from build123d import *

# Parameters (mm, degrees)
BASIC_SHAPE_DEPTH              = 4.9
SIDE_PROFILE1_DEPTH            = 4.55
SIDE_PROFILE1_DEPTH_BACK       = 4.55
SIDE_PROFILE2_DEPTH            = 4.55
SIDE_PROFILE2_DEPTH_BACK       = 4.55
LOCATION_MARK_DEPTH            = 0.8
SKETCH6_W                      = 0.25
SKETCH6_H                      = 1.39
PIN_RELIEF_DEPTH               = 1.25
REMAINING_PINS_COUNT           = 4
REMAINING_PINS_PITCH           = 2.54
REMAINING_PINS_COPY_1_SKETCH_W = 0.25
REMAINING_PINS_COPY_1_SKETCH_H = 1.39
REMAINING_PINS_COPY_2_SKETCH_W = 0.25
REMAINING_PINS_COPY_2_SKETCH_H = 1.39
REMAINING_PINS_COPY_3_SKETCH_W = 0.25
REMAINING_PINS_COPY_3_SKETCH_H = 1.39
REMAINING_PINS_COPY_4_DEPTH    = 1.25
REMAINING_PINS_COPY_5_DEPTH    = 1.25
REMAINING_PINS_COPY_6_DEPTH    = 1.25
PIN_SHAPE1_DEPTH               = 0.445
PIN_START                      = -0.445
PIN_SHAPE2_DEPTH               = 0.445


with BuildPart() as part:
    # Sketch1 → Basic Shape (new body, symmetric)
    with BuildSketch(Plane(origin=(0, 0, 0), x_dir=(1, 0, 0), z_dir=(0, 1, 0))):
        Polygon((-3.3, -0.7), (-3.55, -2.75), (-3.3, -4.8), (3.3, -4.8), (3.55, -2.75), (3.3, -0.7), align=None)
    extrude(amount=BASIC_SHAPE_DEPTH, both=True)

    # Sketch2 → Side Profile1 (cut, two sides)
    with BuildSketch(Plane(origin=(0, 0, 0), x_dir=(0, 0, -1), z_dir=(1, 0, 0))) as side_profile1_sk:
        Polygon((-4.8, 4.9), (-4.8, 4.65), (-2.75, 4.9), align=None)
        Polygon((-4.8, -4.9), (-2.75, -4.9), (-4.8, -4.65), align=None)
    extrude(amount=SIDE_PROFILE1_DEPTH, mode=Mode.SUBTRACT)
    extrude(side_profile1_sk.sketch, amount=-SIDE_PROFILE1_DEPTH_BACK, mode=Mode.SUBTRACT)

    # Sketch3 → Side Profile2 (cut, two sides)
    with BuildSketch(Plane(origin=(0, 0, 0), x_dir=(0, 0, -1), z_dir=(1, 0, 0))) as side_profile2_sk:
        Polygon((-2.75, 4.9), (-0.7, 4.9), (-0.7, 4.65), align=None)
        Polygon((-2.75, -4.9), (-0.7, -4.9), (-0.7, -4.65), align=None)
    extrude(amount=SIDE_PROFILE2_DEPTH, mode=Mode.SUBTRACT)
    extrude(side_profile2_sk.sketch, amount=-SIDE_PROFILE2_DEPTH_BACK, mode=Mode.SUBTRACT)

    # Sketch4 → Location Mark (cut)
    with BuildSketch(Plane(origin=(0, 0, 4.8), x_dir=(-1, 0, 0), z_dir=(0, 0, -1))):
        with BuildLine():
            Line((0.7, 4.65), (0.7, 3.45))
            ThreePointArc((0.7, 3.45), (0, 2.75), (-0.7, 3.45))
            Line((-0.7, 3.45), (-0.7, 4.65))
            Line((-0.7, 4.65), (0.7, 4.65))
        make_face()
    extrude(amount=LOCATION_MARK_DEPTH, mode=Mode.SUBTRACT)

    # First Pin: sweep along a path in Sketch5
    with BuildLine(Plane(origin=(0, -3.9, 0), x_dir=(1, 0, 0), z_dir=(0, 1, 0))) as first_pin_path:
        Line((0, -2.75), (3.31, -2.75))
        ThreePointArc((3.31, -2.75), (3.663553391, -2.603553391), (3.81, -2.25))
        Line((3.81, -2.25), (3.81, 3.3))
    # Sketch6 → First Pin (sweep)
    with BuildSketch(Plane(origin=(0, 0, 0), x_dir=(0, 0, -1), z_dir=(1, 0, 0))):
        with Locations((-2.75, -3.9)):
            Rectangle(SKETCH6_W, SKETCH6_H)
    first_pin = sweep(path=first_pin_path.line)

    # Sketch7 → Pin Relief (cut, through all)
    with BuildSketch(Plane.ZY.offset(-3.685)):
        Polygon((-3.3, -4.15), (0, -4.15), (0, -4.3725), (0.7, -4.595), (-3.3, -4.595), align=None)
        Polygon((-3.3, -3.65), (0, -3.65), (0, -3.4275), (0.7, -3.205), (-3.3, -3.205), align=None)
    pin_relief = extrude(amount=-PIN_RELIEF_DEPTH, mode=Mode.SUBTRACT)

    # Opp Pin: First Pin, Pin Relief across plane
    add(first_pin.mirror(Plane(origin=(0, 0, 0), x_dir=(0, 0, 1), z_dir=(1, 0, 0))))
    add(pin_relief.mirror(Plane(origin=(0, 0, 0), x_dir=(0, 0, 1), z_dir=(1, 0, 0))), mode=Mode.SUBTRACT)

    # Remaining Pins: First Pin, Pin Relief ×4
    with Locations(*[(0, i * REMAINING_PINS_PITCH, 0) for i in range(1, REMAINING_PINS_COUNT)]):
        add(first_pin)
        add(pin_relief, mode=Mode.SUBTRACT)

    # Remaining Pins copy 1: sweep along a path in Remaining Pins copy 1 path
    with BuildLine(Plane(origin=(0, -1.36, 0), x_dir=(-1, 0, 0), z_dir=(0, 1, 0))) as remaining_pins_copy_1_path:
        Line((0, 2.75), (3.31, 2.75))
        ThreePointArc((3.31, 2.75), (3.663553391, 2.603553391), (3.81, 2.25))
        Line((3.81, 2.25), (3.81, -3.3))
    # Remaining Pins copy 1 sketch → Remaining Pins copy 1 (sweep)
    with BuildSketch(Plane(origin=(0, 2.54, 0), x_dir=(0, 0, -1), z_dir=(-1, 0, 0))):
        with Locations((-2.75, 3.9)):
            Rectangle(REMAINING_PINS_COPY_1_SKETCH_W, REMAINING_PINS_COPY_1_SKETCH_H)
    sweep(path=remaining_pins_copy_1_path.line)

    # Remaining Pins copy 2: sweep along a path in Remaining Pins copy 2 path
    with BuildLine(Plane(origin=(0, 1.18, 0), x_dir=(-1, 0, 0), z_dir=(0, 1, 0))) as remaining_pins_copy_2_path:
        Line((0, 2.75), (3.31, 2.75))
        ThreePointArc((3.31, 2.75), (3.663553391, 2.603553391), (3.81, 2.25))
        Line((3.81, 2.25), (3.81, -3.3))
    # Remaining Pins copy 2 sketch → Remaining Pins copy 2 (sweep)
    with BuildSketch(Plane(origin=(0, 5.08, 0), x_dir=(0, 0, -1), z_dir=(-1, 0, 0))):
        with Locations((-2.75, 3.9)):
            Rectangle(REMAINING_PINS_COPY_2_SKETCH_W, REMAINING_PINS_COPY_2_SKETCH_H)
    sweep(path=remaining_pins_copy_2_path.line)

    # Remaining Pins copy 3: sweep along a path in Remaining Pins copy 3 path
    with BuildLine(Plane(origin=(0, 3.72, 0), x_dir=(-1, 0, 0), z_dir=(0, 1, 0))) as remaining_pins_copy_3_path:
        Line((0, 2.75), (3.31, 2.75))
        ThreePointArc((3.31, 2.75), (3.663553391, 2.603553391), (3.81, 2.25))
        Line((3.81, 2.25), (3.81, -3.3))
    # Remaining Pins copy 3 sketch → Remaining Pins copy 3 (sweep)
    with BuildSketch(Plane(origin=(0, 7.62, 0), x_dir=(0, 0, -1), z_dir=(-1, 0, 0))):
        with Locations((-2.75, 3.9)):
            Rectangle(REMAINING_PINS_COPY_3_SKETCH_W, REMAINING_PINS_COPY_3_SKETCH_H)
    sweep(path=remaining_pins_copy_3_path.line)

    # Remaining Pins copy 4 sketch → Remaining Pins copy 4 (cut, through all)
    with BuildSketch(Plane(origin=(-3.685, 2.54, 0), x_dir=(0, 0, 1), z_dir=(1, 0, 0))):
        Polygon((-3.3, 4.15), (0, 4.15), (0, 4.3725), (0.7, 4.595), (-3.3, 4.595), align=None)
        Polygon((-3.3, 3.65), (0, 3.65), (0, 3.4275), (0.7, 3.205), (-3.3, 3.205), align=None)
    extrude(amount=-REMAINING_PINS_COPY_4_DEPTH, mode=Mode.SUBTRACT)

    # Remaining Pins copy 5 sketch → Remaining Pins copy 5 (cut, through all)
    with BuildSketch(Plane(origin=(-3.685, 5.08, 0), x_dir=(0, 0, 1), z_dir=(1, 0, 0))):
        Polygon((-3.3, 4.15), (0, 4.15), (0, 4.3725), (0.7, 4.595), (-3.3, 4.595), align=None)
        Polygon((-3.3, 3.65), (0, 3.65), (0, 3.4275), (0.7, 3.205), (-3.3, 3.205), align=None)
    extrude(amount=-REMAINING_PINS_COPY_5_DEPTH, mode=Mode.SUBTRACT)

    # Remaining Pins copy 6 sketch → Remaining Pins copy 6 (cut, through all)
    with BuildSketch(Plane(origin=(-3.685, 7.62, 0), x_dir=(0, 0, 1), z_dir=(1, 0, 0))):
        Polygon((-3.3, 4.15), (0, 4.15), (0, 4.3725), (0.7, 4.595), (-3.3, 4.595), align=None)
        Polygon((-3.3, 3.65), (0, 3.65), (0, 3.4275), (0.7, 3.205), (-3.3, 3.205), align=None)
    extrude(amount=-REMAINING_PINS_COPY_6_DEPTH, mode=Mode.SUBTRACT)

    # Sketch9 → Pin Shape1 (cut)
    with BuildSketch(Plane.XZ.offset(4.595)):
        with BuildLine():
            Line((3.935, 0), (3.685, 0))
            Line((3.685, 0), (3.685, 2.25))
            ThreePointArc((3.685, 2.25), (3.642990838, 2.422458987), (3.526375455, 2.556278733))
            Line((3.526375455, 2.556278733), (3.55, 2.75))
            Line((3.55, 2.75), (3.540110055, 2.83109755))
            ThreePointArc((3.540110055, 2.83109755), (3.826935095, 2.601287785), (3.935, 2.25))
            Line((3.935, 2.25), (3.935, 0))
        make_face()
        with BuildLine():
            Line((-3.935, 0), (-3.685, 0))
            Line((-3.685, 0), (-3.685, 2.25))
            ThreePointArc((-3.685, 2.25), (-3.642990838, 2.422458987), (-3.526375455, 2.556278733))
            Line((-3.526375455, 2.556278733), (-3.55, 2.75))
            Line((-3.55, 2.75), (-3.540110055, 2.83109755))
            ThreePointArc((-3.540110055, 2.83109755), (-3.826935095, 2.601287785), (-3.935, 2.25))
            Line((-3.935, 2.25), (-3.935, 0))
        make_face()
    extrude(amount=-PIN_SHAPE1_DEPTH, mode=Mode.SUBTRACT)

    # Sketch10 → Pin Shape2 (cut)
    with BuildSketch(Plane(origin=(0, 4.415, 0), x_dir=(-1, 0, 0), z_dir=(0, 1, 0)).offset(PIN_START)):
        with BuildLine():
            Line((-3.935, 0), (-3.685, 0))
            Line((-3.685, 0), (-3.685, 2.25))
            ThreePointArc((-3.685, 2.25), (-3.642990838, 2.422458987), (-3.526375455, 2.556278733))
            Line((-3.526375455, 2.556278733), (-3.55, 2.75))
            Line((-3.55, 2.75), (-3.540110055, 2.83109755))
            ThreePointArc((-3.540110055, 2.83109755), (-3.826935095, 2.601287785), (-3.935, 2.25))
            Line((-3.935, 2.25), (-3.935, 0))
        make_face()
        with BuildLine():
            Line((3.935, 0), (3.685, 0))
            Line((3.685, 0), (3.685, 2.25))
            ThreePointArc((3.685, 2.25), (3.642990838, 2.422458987), (3.526375455, 2.556278733))
            Line((3.526375455, 2.556278733), (3.55, 2.75))
            Line((3.55, 2.75), (3.540110055, 2.83109755))
            ThreePointArc((3.540110055, 2.83109755), (3.826935095, 2.601287785), (3.935, 2.25))
            Line((3.935, 2.25), (3.935, 0))
        make_face()
    extrude(amount=PIN_SHAPE2_DEPTH, mode=Mode.SUBTRACT)


solid = part.part
Design review of the part built by this model. Coordinates are the model's own, in mm. A direction names the side the tool comes from. Round coordinates to 2 decimals unless told otherwise and drop trailing zeros. Order: outer loops, then holes, each group sorted by start corner. A loop starts at its lowest first (then second) coordinate and runs counter-clockwise, first axis right, second up.
1) Consider section A-A (z = -0.75). Count the separate pieces of the cut face and the enclosed holes in it, plus the area to 3 significant figures.
The answers:
separate pieces: 8
enclosed holes: 0
area: 1.00 mm2
2) Consider section D-D (z = 4.25). State the section outline as (x, y) points.
The answers:
outline: (-3.37, -4.72) - (3.37, -4.72) - (3.37, 4.72) - (-3.37, 4.72) - close; hole (-0.7, 3.45) arc R0.7 ccw to (0.7, 3.45) - (0.7, 4.65) - (-0.7, 4.65) - close
3) Consider section C-C (x = 0). State the section outline as (y, z) points.
The answers:
outline: (-4.9, 2.75) - (-4.65, 0.7) - (4.65, 0.7) - (4.9, 2.75) - (4.65, 4.8) - (4.65, 4) - (2.75, 4) - (2.75, 4.8) - (-4.65, 4.8) - close
4) Consider section B-B (y = 3.75). State the section outline as (x, z) points (3 decimals).
The answers:
outline: (-3.935, -3.3) - (-3.685, -3.3) - (-3.685, 2.25) arc R0.375 cw to (-3.526, 2.556) - (-3.3, 0.7) - (3.3, 0.7) - (3.526, 2.556) arc R0.375 cw to (3.685, 2.25) - (3.685, -3.3) - (3.935, -3.3) - (3.935, 2.25) arc R0.625 ccw to (3.54, 2.831) - (3.3, 4.8) - (0.7, 4.8) - (0.7, 4) - (-0.7, 4) - (-0.7, 4.8) - (-3.3, 4.8) - (-3.54, 2.831) arc R0.625 ccw to (-3.935, 2.25) - close
5) For L1, parallel to X at y = -3.5, z = 2 (3 decimals); L2, parallel to Z at x = 2.5, y = -2.25; L3, parallel to X at y = -4, z = 0.5 (3 decimals), list the stretches that pass through material, from the lowest coordinate up.
The answers:
L1: x = -3.935 to -3.685, -3.459 to 3.459, 3.685 to 3.935
L2: z = 0.7 to 4.8
L3: x = -3.935 to -3.685, 3.685 to 3.935
6) Clearance check with flat-ended pins moving along their axes: pin 1 Ø0.6 at (x, z) = (-0.5, 4.5) entering from -Y; pin 2 Ø0.6 at (y, z) = (4, 4.5) entering from -X; pin 3 Ø3 at (x, z) = (-3, 1) entering from -Y; pin 4 Ø3 at (x, z) = (-1.5, -1.5) entering from +Y. State where each tip first meets the part, or that it passes through.
The answers:
pin 1: stops at y = -4.72
pin 2: stops at x = -3.37
pin 3: stops at y = -4.87
pin 4: passes through
7) Draft analysis for pull direction X (two halves, no side actions). For faces 1 (the flat face through (3.685, 1.2, 0.1)), 2 (the flat face through (0, 0, 4.8)), 3 (the flat face through (3.935, 1.2, 0.1)), 4 (the flat face through (-3.935, 1.2, 0.1)), state which applies: released by +X, released by -X, zero draft, split by the parting line, or undercut.
The answers:
face 1: undercut
face 2: zero draft
face 3: released by +X
face 4: released by -X
8) Machinability: for faces 5 (the flat face through (3.935, 3.6, 0.1)), 6 (the flat face through (-3.685, -3.8, 0.1)), which of the approach directions +Z, -Z, +X, -X, +Y, -Y give a long, thin tool a straight path to every point of the face, cutting with its end or side? Answer none if there is none.
The answers:
face 5: +Z, -Z, +X, +Y, -Y
face 6: -Z, +Y, -Y
